from build123d import *

# Parameters (mm, degrees)
SKETCH1_R               = 150
BOSS_EXTRUDE1_DEPTH     = 150
SKETCH2_W               = 190
SKETCH2_H               = 190
CUT_EXTRUDE1_DEPTH      = 150
CUT_EXTRUDE2_DEPTH      = 260.807621135
CUT_EXTRUDE2_DEPTH_BACK = 260.807621135
SKETCH3_R               = 43
CUT_EXTRUDE3_DEPTH      = 260.807621309
CUT_EXTRUDE3_DEPTH_BACK = 260.807621309
SKETCH4_R               = 43


with BuildPart() as part:
    # Sketch1 → Boss-Extrude1 (new body)
    with BuildSketch(Plane(origin=(0, 0, 0), x_dir=(1, 0, 0), z_dir=(0, 1, 0))):
        with Locations(Location((0, 0, 0), (0, 0, 270))):
            Circle(SKETCH1_R)
    extrude(amount=BOSS_EXTRUDE1_DEPTH)

    # Sketch2 → Cut-Extrude1 (cut)
    with BuildSketch(Plane(origin=(0, 150, 0), x_dir=(1, 0, 0), z_dir=(0, 1, 0))):
        Rectangle(SKETCH2_W, SKETCH2_H)
    extrude(amount=-CUT_EXTRUDE1_DEPTH, mode=Mode.SUBTRACT)

    # Sketch3 → Cut-Extrude2 (cut, two sides: drawn at the far end of the back side and taken through both)
    with BuildSketch(Plane.XY.offset(-CUT_EXTRUDE2_DEPTH_BACK)):
        with Locations((0, 75)):
            Circle(SKETCH3_R)
    extrude(amount=CUT_EXTRUDE2_DEPTH + CUT_EXTRUDE2_DEPTH_BACK, mode=Mode.SUBTRACT)

    # Sketch4 → Cut-Extrude3 (cut, two sides: drawn at the far end of the back side and taken through both)
    with BuildSketch(Plane(origin=(0, 0, 0), x_dir=(0, 0, -1), z_dir=(1, 0, 0)).offset(-CUT_EXTRUDE3_DEPTH_BACK)):
        with Locations((0, 75)):
            Circle(SKETCH4_R)
    extrude(amount=CUT_EXTRUDE3_DEPTH + CUT_EXTRUDE3_DEPTH_BACK, mode=Mode.SUBTRACT)


solid = part.part
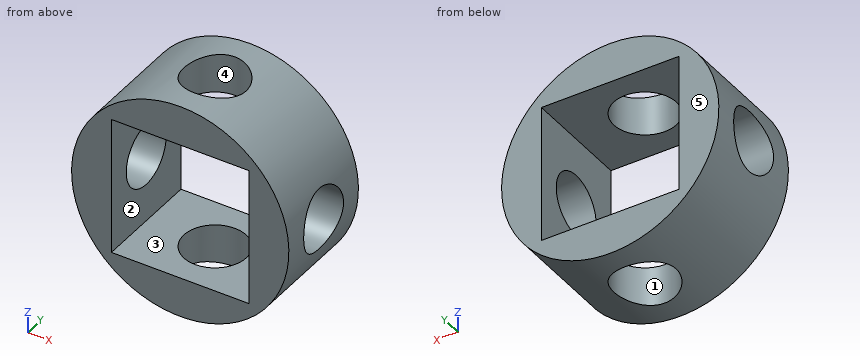
Work out the finished part from the listing and answer in its coordinate system (mm). Face numbers are marked on the shaded views. A direction names the side the tool comes from. Give positions to 0.01 mm unless a question says otherwise; leave off trailing zeros. Order: outer loops, then holes, each group sorted by start corner. A loop starts at its lowest first (then second) coordinate and runs counter-clockwise, first axis right, second up. Notation, with made-up numbers: (-12.75, 12) -> (36.25, 12) arc R23 ccw to (36.25, 38) -> close; hole circle Ø11 at (16, 14). An arc over 180 degrees is marked (long way). Answer as a JSON object with one key per item and string values. Group by question number.
1. Consider line 1 along Y through (x, z) = (-136.5, 0); line 2 along X through (y, z) = (138, 49.5); line 3 along Z through (x, y) = (-116, 75). Determine where each line is inside the solid, lowest interval first. Write a range as [from, to].
2. The mould has two halves that part along Y. Classify the marked faces 3, 4 and 5: released by +Y, released by -Y, zero draft, split by the parting line, or undercut.
3. Section C-C on y = 75 is taken. Determine the outline of the cut face in (x, z), plus the area to 3 significant figures.
4. A tool of negligible diameter and unlimited length cuts with its end or side. For the marked faces 1 and 2, from which of +Z, -Z, +X, -X, +Y, -Y can it reach the whole face along a straight path? Write none if from no direction.
5. Section D-D on y = 136 is taken. Determine the outline of the cut face in (x, z), plus the area to 3 significant figures.
6. Flat-ended cylindrical pins translate along their axes: pin 1 Ø12 at (x, y) = (77, 58) entering from -Z; pin 2 Ø1 at (y, z) = (40, 71.5) entering from -X; pin 3 Ø8 at (x, y) = (-117, 97.5) entering from -Z. Find the tip coordinate at first contact, or state that the pin passes through.
7. Section B-B on x = 0 is taken. Determine the outline of the cut face in (y, z).
8. Section A-A on z = 0 is taken. Determine the outline of the cut face in (x, y), plus the area to 3 significant figures.
Result sheet:
{
 "1": {"line 1": "y = [0, 32], [118, 150]", "line 2": "x = [-141.6, -95], [95, 141.6]", "line 3": "z = [-95.1, -43], [43, 95.1]"},
 "2": {"face 3": "zero draft", "face 4": "undercut", "face 5": "released by +Y"},
 "3": {"outline": "(-143.7, -43) arc R150 ccw to (-43, -143.7) -> (-43, -95) -> (-95, -95) -> (-95, -43) -> close; (-143.7, 43) -> (-95, 43) -> (-95, 95) -> (-43, 95) -> (-43, 143.7) arc R150 ccw to start; (43, -143.7) arc R150 ccw to (143.7, -43) -> (95, -43) -> (95, -95) -> (43, -95) -> close; (43, 95) -> (95, 95) -> (95, 43) -> (143.7, 43) arc R150 ccw to (43, 143.7) -> close", "area": "16,400 mm^2"},
 "4": {"face 1": "+Z, -Z", "face 2": "+Y, -Y"},
 "5": {"outline": "circle Ø300 at (0, 0); hole (-95, -95) -> (95, -95) -> (95, 95) -> (-95, 95) -> close", "area": "34,600 mm^2"},
 "6": {"pin 1": "stops at z = -132.13", "pin 2": "stops at x = -132.13", "pin 3": "stops at z = -98.65"},
 "7": {"outline": "(0, -150) -> (32, -150) -> (32, -95) -> (0, -95) -> close; (0, 95) -> (32, 95) -> (32, 150) -> (0, 150) -> close; (118, -150) -> (150, -150) -> (150, -95) -> (118, -95) -> close; (118, 95) -> (150, 95) -> (150, 150) -> (118, 150) -> close"},
 "8": {"outline": "(-150, 0) -> (-95, 0) -> (-95, 32) -> (-150, 32) -> close; (-150, 118) -> (-95, 118) -> (-95, 150) -> (-150, 150) -> close; (95, 0) -> (150, 0) -> (150, 32) -> (95, 32) -> close; (95, 118) -> (150, 118) -> (150, 150) -> (95, 150) -> close", "area": "7,040 mm^2"}
}
